Source: CAD feature listing. Evaluate the final solid. Frame: model axes, mm. Face numbers are marked on the shaded views. Round coordinates to 2 decimals unless told otherwise and drop trailing zeros. Loops run counter-clockwise (first coordinate to the right, second up) from the corner with the lowest first, then second, coordinate; pieces in that order, holes last. Notation, with made-up numbers: (13, -6) - (66, -6) arc R17 ccw to (66, 13) - close; hole circle Ø8 at (76, 88). An arc over 180 degrees is marked (long way). One line per question, with ' | ' between items. Start each with the question number.
1. Mould query, pull axis Y, two halves, no side actions, for the marked faces 1, 2 and 3. Classes: pulls with the +Y half, pulls with the -Y half, needs draft (parallel to the pull), parting line crosses it, or undercut.
2. Cut plane A-A (y = -17). Return loops of the section in (x, z).
3. Cut plane B-B (y = 15). Return loops of the section in (x, z), then the cut area to 3 significant figures.
4. Cut plane C-C (z = 8.25). Return loops of the section in (x, y), then the cut area to 3 significant figures.
5. Cut plane D-D (x = -14). Return loops of the section in (y, z).
6. Ray query, line 1 (X direction, y = -57, z = 4.75); line 2 (X direction, y = -17, z = 9.5); line 3 (Y direction, x = -11, z = 9). Return the intervals inside material, ascending.
7. Pin query (flat end, axial travel): pin 1 (2.5 mm diameter, centred on x = 45, y = -17, fed in from -Z). Return the tip coordinate at first contact, or that it passes through.
```python
from build123d import *

# Parameters (mm, degrees)
SKETCH1_W               = 110
SKETCH1_H               = 130
BOSS_EXTRUDE1_DEPTH     = 12
CUT_EXTRUDE1_DEPTH      = 86.988371307
CUT_EXTRUDE1_DEPTH_BACK = 86.988371307
SKETCH2_R               = 2
SKETCH3_R               = 21
CUT_EXTRUDE2_DEPTH      = 86.988371307


with BuildPart() as part:
    # Sketch1 → Boss-Extrude1 (new body)
    with BuildSketch(Plane.XY):
        Rectangle(SKETCH1_W, SKETCH1_H)
    extrude(amount=BOSS_EXTRUDE1_DEPTH)

    # Sketch2 → Cut-Extrude1 (cut, two sides: drawn at the far end of the back side and taken through both)
    with BuildSketch(Plane(origin=(0, 0, 0), x_dir=(-1, 0, 0), z_dir=(0, 0, -1)).offset(-CUT_EXTRUDE1_DEPTH_BACK)):
        with Locations((-45, 55)):
            Circle(SKETCH2_R)
        with Locations((-45, -17)):
            Circle(SKETCH2_R)
        with Locations((-47, -57)):
            Circle(SKETCH2_R)
        with Locations((47, -57)):
            Circle(SKETCH2_R)
        with Locations((45, -17)):
            Circle(SKETCH2_R)
        with Locations((45, 55)):
            Circle(SKETCH2_R)
    extrude(amount=CUT_EXTRUDE1_DEPTH + CUT_EXTRUDE1_DEPTH_BACK, mode=Mode.SUBTRACT)

    # Sketch3 → Cut-Extrude2 (cut, through all)
    with BuildSketch(Plane.XY.offset(12)):
        with Locations((0, 15)):
            Circle(SKETCH3_R)
    extrude(amount=-CUT_EXTRUDE2_DEPTH, mode=Mode.SUBTRACT)


solid = part.part
```
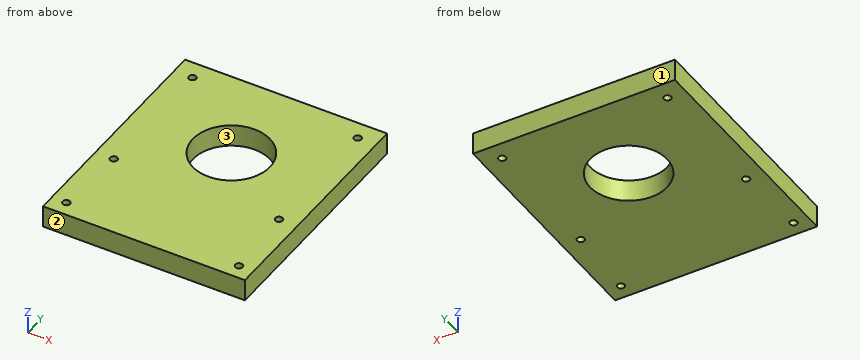
Answers follow:
1) face 1: pulls with the +Y half | face 2: pulls with the -Y half | face 3: undercut
2) outline: (-55, 0) - (-47, 0) - (-47, 12) - (-55, 12) - close; (-43, 0) - (43, 0) - (43, 12) - (-43, 12) - close; (47, 0) - (55, 0) - (55, 12) - (47, 12) - close
3) outline: (-55, 0) - (-21, 0) - (-21, 12) - (-55, 12) - close; (21, 0) - (55, 0) - (55, 12) - (21, 12) - close | area: 816 mm2
4) outline: (-55, -65) - (55, -65) - (55, 65) - (-55, 65) - close; hole circle Ø4 at (-47, -57); hole circle Ø4 at (-45, -17); hole circle Ø4 at (-45, 55); hole circle Ø42 at (0, 15); hole circle Ø4 at (45, -17); hole circle Ø4 at (45, 55); hole circle Ø4 at (47, -57) | area: 12,800 mm2
5) outline: (-65, 0) - (-0.65, 0) - (-0.65, 12) - (-65, 12) - close; (30.65, 0) - (65, 0) - (65, 12) - (30.65, 12) - close
6) line 1: x = -55 to -49, -45 to 45, 49 to 55 | line 2: x = -55 to -47, -43 to 43, 47 to 55 | line 3: y = -65 to -2.89, 32.89 to 65
7) pin 1: passes through
